```python
from build123d import *

# Parameters (mm, degrees)
SKETCH10_W          = 60
SKETCH10_H          = 72.75
SKETCH10_R          = 3.25
SKETCH10_R_2        = 8.5
BOSS_EXTRUDE1_DEPTH = 10
FILLET1_R           = 10


with BuildPart() as part:
    # Sketch10 → Boss-Extrude1 (new body)
    with BuildSketch(Plane(origin=(0, 0, 0), x_dir=(1, 0, 0), z_dir=(0, 1, 0))):
        with Locations((30, 36.375)):
            Rectangle(SKETCH10_W, SKETCH10_H)
        with Locations(Location((10, 57.75, 0), (0, 0, 270))):
            Circle(SKETCH10_R, mode=Mode.SUBTRACT)
        with Locations(Location((17.5, 15, 0), (0, 0, 270))):
            Circle(SKETCH10_R_2, mode=Mode.SUBTRACT)
        with Locations(Location((50, 57.75, 0), (0, 0, 270))):
            Circle(SKETCH10_R, mode=Mode.SUBTRACT)
        with Locations(Location((42.5, 15, 0), (0, 0, 270))):
            Circle(SKETCH10_R_2, mode=Mode.SUBTRACT)
    extrude(amount=BOSS_EXTRUDE1_DEPTH)

    # Fillet1
    fillet1_edges = [part.edges().sort_by_distance(p)[0] for p in [
        (60, 5, 0),
        (0, 5, 0),
    ]]
    fillet(fillet1_edges, radius=FILLET1_R)


solid = part.part
```
Work out the finished part from the listing and answer in its coordinate system (mm). Give positions to 0.01 mm unless a question says otherwise; leave off trailing zeros. Write each loop counter-clockwise with the first axis right and the second up, starting at its lowest first coordinate (ties: lowest second). Pieces come first, ordered by that corner, then holes. Notation, with made-up numbers: (3.25, 83.25) -> (53.25, 83.25) arc R31 cw to (53.25, 107.25) -> close; hole circle Ø6 at (51.5, 41.5). An arc over 180 degrees is marked (long way). Write item = value, one per line.
Q1. Section D-D on z = -14 is taken. Determine the outline of the cut face in (x, y), and give its area (3 significant figures).
Computed values:
outline = (0, 0) -> (9.06, 0) -> (9.06, 10) -> (0, 10) -> close; (25.94, 0) -> (34.06, 0) -> (34.06, 10) -> (25.94, 10) -> close; (50.94, 0) -> (60, 0) -> (60, 10) -> (50.94, 10) -> close
area = 262 mm^2
Q2. For a pull along X with two mould halves and no side action, classify faces 1 (the cylindrical face through (48.022, 4.93, -60.329)), 2 (the flat face through (60, 5, -41)), 3 (the flat face through (30, 5, -72.75)) as pulls with the +X half, pulls with the -X half, needs draft (parallel to the pull), parting line crosses it, or undercut.
Computed values:
face_1 = undercut
face_2 = pulls with the +X half
face_3 = needs draft
Q3. Section A-A on y = 7.25 is taken. Determine the outline of the cut face in (x, z).
Computed values:
outline = (0, -72.75) -> (60, -72.75) -> (60, -10) arc R10 ccw to (50, 0) -> (10, 0) arc R10 ccw to (0, -10) -> close; hole circle Ø6.5 at (10, -57.75); hole circle Ø17 at (17.5, -15); hole circle Ø17 at (42.5, -15); hole circle Ø6.5 at (50, -57.75)
Q4. Section C-C on z = -57.75 is taken. Determine the outline of the cut face in (x, y).
Computed values:
outline = (0, 0) -> (6.75, 0) -> (6.75, 10) -> (0, 10) -> close; (13.25, 0) -> (46.75, 0) -> (46.75, 10) -> (13.25, 10) -> close; (53.25, 0) -> (60, 0) -> (60, 10) -> (53.25, 10) -> close
Q5. Section B-B on x = 17.5 is taken. Determine the outline of the cut face in (y, z), and give its area (4 significant figures).
Computed values:
outline = (0, -72.75) -> (10, -72.75) -> (10, -23.5) -> (0, -23.5) -> close; (0, -6.5) -> (10, -6.5) -> (10, 0) -> (0, 0) -> close
area = 557.5 mm^2
Q6. Consider line 1 along X through (y, z) = (7, -15); line 2 along X through (y, z) = (7, -57.75); line 3 along Z through (x, y) = (12.5, 8.25). Determine where each line is inside the solid, lowest interval first.
Computed values:
line_1 = 0 to 9, 26 to 34, 51 to 60
line_2 = 0 to 6.75, 13.25 to 46.75, 53.25 to 60
line_3 = -72.75 to -59.83, -55.67 to -21.87, -8.13 to 0
Q7. Flat-ended cylindrical pins translate along their axes: pin 1 Ø22 at (x, z) = (17.5, -15) entering from +Y; pin 2 Ø15.5 at (x, z) = (42.5, -15) entering from +Y; pin 3 Ø1.5 at (x, y) = (52, 6.5) entering from +Z. Find the tip coordinate at first contact, or state that the pin passes through.
Computed values:
pin_1 = 10
pin_2 = through
pin_3 = -0.08
